Geometry: final body of the model. Coordinates: model frame, mm. Face numbers are marked on the shaded views. Give positions to 0.01 mm unless a question says otherwise; leave off trailing zeros. Write each loop counter-clockwise with the first axis right and the second up, starting at its lowest first coordinate (ties: lowest second). Pieces come first, ordered by that corner, then holes.
Q1. Cut plane A-A on x = -6. Return the cut outline in (y, z), plus the area to 3 significant figures.
Q2. Draft query along X for the marked faces 1, 2 and 3. Return one class per face: pulls with the +X half, pulls with the -X half, needs draft (parallel to the pull), parting line crosses it, or undercut.
Q3. Cut plane D-D on z = 15.5. Return the cut outline in (x, y), plus the area to 3 significant figures.
Q4. Cut plane B-B on y = 64. Return the cut outline in (x, z), plus the area to 3 significant figures.
Q5. Cut plane C-C on z = 0. Count the separate pieces of the cut face and the enclosed holes in it, plus the area to 3 significant figures.
Q6. Line query: L1, parallel to Y at x = 7, z = 12.5; L2, parallel to X at y = 150.95, z = 0; L3, parallel to Y at x = -0.5, z = 6. Output: solid intervals per line, ascending.
Q7. Pin query (flat end, axial travel): pin 1 (10 mm diameter, centred on x = 8, y = 184, fed in from +Z); pin 2 (2.5 mm diameter, centred on x = 10, z = 0, fed in from +Y); pin 3 (1.5 mm diameter, centred on x = 14, y = 123.5, fed in from -Z). Return the tip coordinate at first contact, or that it passes through.
```python
from build123d import *

# Parameters (mm, degrees)
SKETCH_1_R      = 19
SKETCH_1_R_2    = 18
EXTRUDE_1_DEPTH = 150
SKETCH_2_R      = 19
SKETCH_2_R_2    = 2
SKETCH_2_R_3    = 2.5
EXTRUDE_2_DEPTH = 2
SKETCH_3_R      = 19
SKETCH_3_R_2    = 18
EXTRUDE_3_DEPTH = 50
SKETCH_4_R      = 19
SKETCH_4_R_2    = 2.5
EXTRUDE_4_DEPTH = 2
SKETCH_5_R      = 3.5
SKETCH_5_R_2    = 2.5
EXTRUDE_5_DEPTH = 10
EXTRUDE_START   = 2
SKETCH_6_R      = 19
SKETCH_6_R_2    = 12.5
EXTRUDE_6_DEPTH = 2


with BuildPart() as part:
    # 草图1 → 凸台-拉伸1 (new body)
    with BuildSketch(Plane(origin=(0, 0, 0), x_dir=(1, 0, 0), z_dir=(0, 1, 0))):
        with Locations(Location((0, 0, 0), (0, 0, 270))):
            Circle(SKETCH_1_R)
        with Locations(Location((0, 0, 0), (0, 0, 270))):
            Circle(SKETCH_1_R_2, mode=Mode.SUBTRACT)
    extrude(amount=EXTRUDE_1_DEPTH)

    # 草图2 → 凸台-拉伸2 (add)
    with BuildSketch(Plane(origin=(0, 150, 0), x_dir=(1, 0, 0), z_dir=(0, 1, 0))):
        with Locations(Location((0, 0, 0), (0, 0, 270))):
            Circle(SKETCH_2_R)
        with Locations(Location((10, 0, 0), (0, 0, 270))):
            Circle(SKETCH_2_R_2, mode=Mode.SUBTRACT)
        with Locations(Location((-10, 0, 0), (0, 0, 270))):
            Circle(SKETCH_2_R_2, mode=Mode.SUBTRACT)
        with Locations(Location((0, -10, 0), (0, 0, 270))):
            Circle(SKETCH_2_R_2, mode=Mode.SUBTRACT)
        with Locations(Location((0, 0, 0), (0, 0, 270))):
            Circle(SKETCH_2_R_3, mode=Mode.SUBTRACT)
        Polygon((0, 10), (0, 15.61), (6.2, 15.61), (6.2, 9.89), (0, 9.89), align=None, mode=Mode.SUBTRACT)
    extrude(amount=EXTRUDE_2_DEPTH)

    # 草图3 → 凸台-拉伸3 (add)
    with BuildSketch(Plane(origin=(0, 152, 0), x_dir=(1, 0, 0), z_dir=(0, 1, 0))):
        with Locations(Location((0, 0, 0), (0, 0, 270))):
            Circle(SKETCH_3_R)
        with Locations(Location((0, 0, 0), (0, 0, 270))):
            Circle(SKETCH_3_R_2, mode=Mode.SUBTRACT)
    extrude(amount=EXTRUDE_3_DEPTH)

    # 草图4 → 凸台-拉伸4 (add)
    with BuildSketch(Plane(origin=(0, 202, 0), x_dir=(1, 0, 0), z_dir=(0, 1, 0))):
        with Locations(Location((0, 0, 0), (0, 0, 270))):
            Circle(SKETCH_4_R)
        with Locations(Location((0, 0, 0), (0, 0, 270))):
            Circle(SKETCH_4_R_2, mode=Mode.SUBTRACT)
    extrude(amount=EXTRUDE_4_DEPTH)

    # 草图5 → 凸台-拉伸5 (add)
    with BuildSketch(Plane(origin=(0, 204, 0), x_dir=(1, 0, 0), z_dir=(0, 1, 0))):
        with Locations(Location((0, 0, 0), (0, 0, 270))):
            Circle(SKETCH_5_R)
        with Locations(Location((0, 0, 0), (0, 0, 270))):
            Circle(SKETCH_5_R_2, mode=Mode.SUBTRACT)
    extrude(amount=EXTRUDE_5_DEPTH)

    # 草图6 → 凸台-拉伸6 (add)
    with BuildSketch(Plane.XZ.offset(EXTRUDE_START)):
        with Locations(Location((0, 0, 0), (0, 0, 270))):
            Circle(SKETCH_6_R)
        with Locations(Location((0, 0, 0), (0, 0, 270))):
            Circle(SKETCH_6_R_2, mode=Mode.SUBTRACT)
    extrude(amount=-EXTRUDE_6_DEPTH)


solid = part.part
```
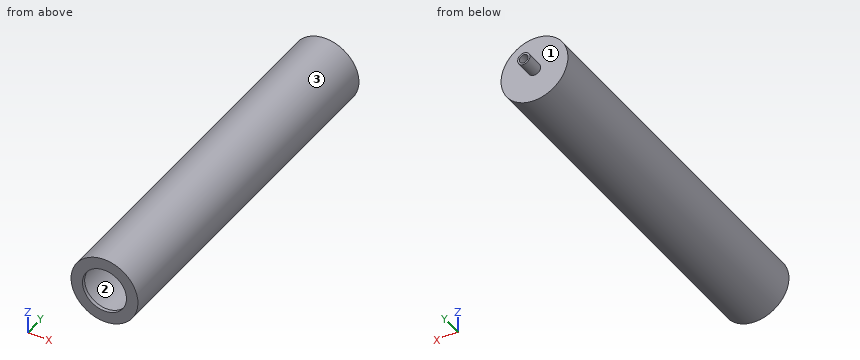
Data:
1. outline: (-2, -18.03) - (204, -18.03) - (204, 18.03) - (-2, 18.03) - (-2, 10.97) - (0, 10.97) - (0, 16.97) - (150, 16.97) - (150, -16.97) - (0, -16.97) - (0, -10.97) - (-2, -10.97) - close; hole (152, -16.97) - (202, -16.97) - (202, 16.97) - (152, 16.97) - close
1. area: 595 mm2
2. face 1: needs draft
2. face 2: undercut
2. face 3: parting line crosses it
3. outline: (-10.99, -2) - (10.99, -2) - (10.99, 204) - (-10.99, 204) - close; hole (-9.15, 0) - (9.15, 0) - (9.15, 150) - (-9.15, 150) - close; hole (-9.15, 152) - (9.15, 152) - (9.15, 202) - (-9.15, 202) - close
3. area: 867 mm2
4. outline: circle Ø38 at (0, 0); hole circle Ø36 at (0, 0)
4. area: 116 mm2
5. separate pieces: 4
5. enclosed holes: 0
5. area: 562 mm2
6. L1: y = -2 to 0, 150 to 152, 202 to 204
6. L2: x = -19 to -12, -8 to -2.5, 2.5 to 8, 12 to 19
6. L3: y = 150 to 152, 202 to 204
7. pin 1: stops at z = 18.76
7. pin 2: stops at y = 204
7. pin 3: stops at z = -13.62
